Design review of the part built by this model. Coordinates are the model's own, in mm. A direction names the side the tool comes from. Round coordinates to 2 decimals unless told otherwise and drop trailing zeros. Order: outer loops, then holes, each group sorted by start corner. A loop starts at its lowest first (then second) coordinate and runs counter-clockwise, first axis right, second up.
from build123d import *

# Parameters (mm, degrees)
F1_DEPTH = 4.4
F3_DEPTH = 1
F4_DEPTH = 1


with BuildPart() as f1:
    # F0 (on Top) → F1 (new body)
    with BuildSketch(Plane.XY):
        with BuildLine():
            ThreePointArc((10.22, 4.625), (9.9271067812, 5.3321067812), (9.22, 5.625))
            Line((9.22, 5.625), (-9.22, 5.625))
            ThreePointArc((-9.22, 5.625), (-9.9271067812, 5.3321067812), (-10.22, 4.625))
            Line((-10.22, 4.625), (-10.22, -4.625))
            ThreePointArc((-10.22, -4.625), (-9.9271067812, -5.3321067812), (-9.22, -5.625))
            Line((-9.22, -5.625), (9.22, -5.625))
            ThreePointArc((9.22, -5.625), (9.9271067812, -5.3321067812), (10.22, -4.625))
            Line((10.22, -4.625), (10.22, 4.625))
        make_face()
        with BuildLine():
            Line((-7.22, 3.625), (7.22, 3.625))
            ThreePointArc((7.22, 3.625), (7.9271067812, 3.3321067812), (8.22, 2.625))
            Line((8.22, 2.625), (8.22, -2.625))
            ThreePointArc((8.22, -2.625), (7.9271067812, -3.3321067812), (7.22, -3.625))
            Line((7.22, -3.625), (-7.22, -3.625))
            ThreePointArc((-7.22, -3.625), (-7.9271067812, -3.3321067812), (-8.22, -2.625))
            Line((-8.22, -2.625), (-8.22, 2.625))
            ThreePointArc((-8.22, 2.625), (-7.9271067812, 3.3321067812), (-7.22, 3.625))
        make_face(mode=Mode.SUBTRACT)
    extrude(amount=F1_DEPTH)

    # F2 (on face) → F3 (join)
    with BuildSketch(Plane.XY.offset(4.4)):
        with BuildLine():
            Line((7.22, 3.625), (-7.22, 3.625))
            ThreePointArc((-7.22, 3.625), (-7.9271067812, 3.3321067812), (-8.22, 2.625))
            Line((-8.22, 2.625), (-8.22, -2.625))
            ThreePointArc((-8.22, -2.625), (-7.9271067812, -3.3321067812), (-7.22, -3.625))
            Line((-7.22, -3.625), (7.22, -3.625))
            ThreePointArc((7.22, -3.625), (7.9271067812, -3.3321067812), (8.22, -2.625))
            Line((8.22, -2.625), (8.22, 2.625))
            ThreePointArc((8.22, 2.625), (7.9271067812, 3.3321067812), (7.22, 3.625))
        make_face()
        with BuildLine():
            ThreePointArc((7.2, -2.05), (7.0242640687, -2.4742640687), (6.6, -2.65))
            Line((6.6, -2.65), (-6.6, -2.65))
            ThreePointArc((-6.6, -2.65), (-7.0242640687, -2.4742640687), (-7.2, -2.05))
            Line((-7.2, -2.05), (-7.2, 2.05))
            ThreePointArc((-7.2, 2.05), (-7.0242640687, 2.4742640687), (-6.6, 2.65))
            Line((-6.6, 2.65), (6.6, 2.65))
            ThreePointArc((6.6, 2.65), (7.0242640687, 2.4742640687), (7.2, 2.05))
            Line((7.2, 2.05), (7.2, -2.05))
        make_face(mode=Mode.SUBTRACT)
    extrude(amount=F3_DEPTH)

    # F4 (add): a face of the model
    f4_faces = [f1.faces().sort_by_distance(p)[0] for p in [
        (9.9866855984, 0, 4.4),
    ]]
    extrude(f4_faces, amount=F4_DEPTH)


solid = f1.part
1) Take a section at C-C on x = 0. Give the boundary of the cut face in (y, z) (3 decimals), plus the area to 4 significant figures.
Results:
outline: (-5.625, 0) - (-3.625, 0) - (-3.625, 4.4) - (-2.65, 4.4) - (-2.65, 5.4) - (-5.625, 5.4) - close; (2.65, 4.4) - (3.625, 4.4) - (3.625, 0) - (5.625, 0) - (5.625, 5.4) - (2.65, 5.4) - close
area: 23.55 mm2
2) Take a section at B-B on z = 4.7. Give the boundary of the cut face in (x, y) (3 decimals).
Results:
outline: (-10.22, -4.625) arc R1 ccw to (-9.22, -5.625) - (9.22, -5.625) arc R1 ccw to (10.22, -4.625) - (10.22, 4.625) arc R1 ccw to (9.22, 5.625) - (-9.22, 5.625) arc R1 ccw to (-10.22, 4.625) - close; hole (-7.2, -2.05) arc R0.6 ccw to (-6.6, -2.65) - (6.6, -2.65) arc R0.6 ccw to (7.2, -2.05) - (7.2, 2.05) arc R0.6 ccw to (6.6, 2.65) - (-6.6, 2.65) arc R0.6 ccw to (-7.2, 2.05) - close
3) The part is to be moulded in two halves that separate along Y. For faces 4 (the face through (-9.92, 5.34, 2.66)), 5 (the face through (0, -5.625, 3)), 6 (the face through (0, 2.65, 5)), say which applies: released by +Y, released by -Y, zero draft, split by the parting line, or undercut.
Results:
face 4: released by +Y
face 5: released by -Y
face 6: undercut
4) For faces 1 (the face through (-7.935, 3.324, 2.169)), 2 (the face through (-7.2, 0, 5)), 3 (the face through (0, 4, 0)), list the 3-axis set-ups (+Z, -Z, +X, -X, +Y, -Y) from which the entire face can be reached by the end or side of a thin tool; tool diameter is ignored.
Results:
face 1: -Z
face 2: +Z, -Z
face 3: -Z, +X, -X, +Y, -Y
5) To check wall thickness, follow line 1 along Y through (x, z) = (-2, 4.15) (3 decimals); line 2 along X through (y, z) = (0, 2.3); line 3 along X through (y, z) = (1, 5.1). State the ranges of each line that lie inside material, in increasing order.
Results:
line 1: y = -5.625 to -3.625, 3.625 to 5.625
line 2: x = -10.22 to -8.22, 8.22 to 10.22
line 3: x = -10.22 to -7.2, 7.2 to 10.22
6) Take a section at A-A on y = 0.25. Give the boundary of the cut face in (x, z).
Results:
outline: (-10.22, 0) - (-8.22, 0) - (-8.22, 4.4) - (-7.2, 4.4) - (-7.2, 5.4) - (-10.22, 5.4) - close; (7.2, 4.4) - (8.22, 4.4) - (8.22, 0) - (10.22, 0) - (10.22, 5.4) - (7.2, 5.4) - close
7) Clearance check with a flat-ended pin moving along its axis: P1, Ø2, axis at x = -2, y = 0, coming from the -Z side. State where the tip first meets the part, or that it passes through.
Results:
P1: passes through
8) Take a section at D-D on z = 3.65. Give the boundary of the cut face in (x, y) (3 decimals), plus the area to 3 significant figures.
Results:
outline: (-10.22, -4.625) arc R1 ccw to (-9.22, -5.625) - (9.22, -5.625) arc R1 ccw to (10.22, -4.625) - (10.22, 4.625) arc R1 ccw to (9.22, 5.625) - (-9.22, 5.625) arc R1 ccw to (-10.22, 4.625) - close; hole (-8.22, -2.625) arc R1 ccw to (-7.22, -3.625) - (7.22, -3.625) arc R1 ccw to (8.22, -2.625) - (8.22, 2.625) arc R1 ccw to (7.22, 3.625) - (-7.22, 3.625) arc R1 ccw to (-8.22, 2.625) - close
area: 111 mm2
